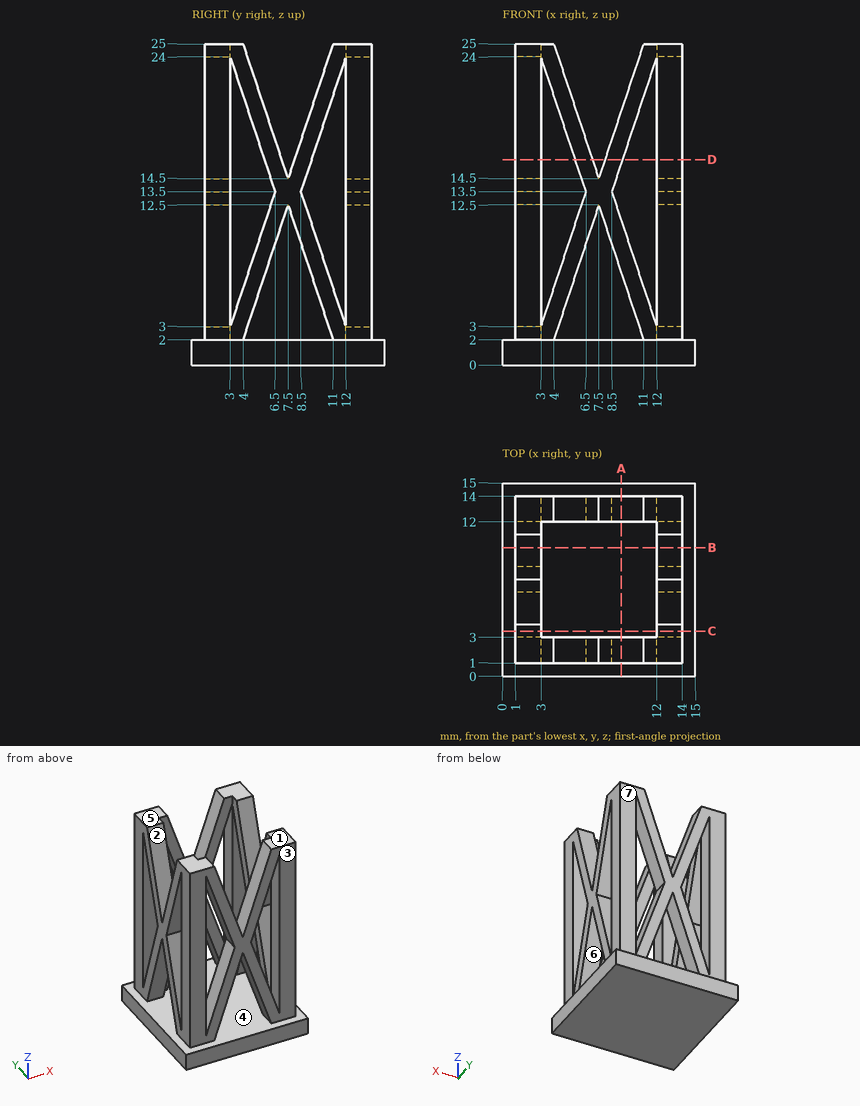
Input: dimensioned drawing with shaded views. Units: mm. Origin: part minimum x, y, z. A direction names the side the tool comes from. Round coordinates to 2 decimals unless told otherwise and drop trailing zeros. Loops run counter-clockwise (first coordinate to the right, second up) from the corner with the lowest first, then second, coordinate; pieces in that order, holes last. Notation, with made-up numbers: (-1, 56) -> (4, 56) arc R35 cw to (4, 88) -> close; hole circle Ø8 at (24, -34). An arc over 180 degrees is marked (long way). Use one line per item in the form item = value. Start each with the question number.
1) Section C-C on y = 3.5. Output: boundary loops of the cut face in (x, z), then the cut area to 3 significant figures.
2) Access query for the marked faces 1, 2, 3 and 4. Directions: +Z, -Z, +X, -X, +Y, -Y. A direction counts if a zero-diameter tool reaches every point of the face in a straight line with its end or side. Return the directions, or none.
3) Draft query along Y for the marked faces 5, 6 and 7. Return one class per face: released by +Y, released by -Y, zero draft, split by the parting line, or undercut.
4) Line query: L1, parallel to Y at x = 6, z = 11.25; L2, parallel to Y at x = 13.5, z = 5.5; L3, parallel to X at y = 2.5, z = 19.75. Output: solid intervals per line, ascending.
5) Section A-A on x = 9.25. Output: boundary loops of the cut face in (y, z).
6) Section D-D on z = 16. Give the number of separate pieces and of enclosed holes in the cut face, then the cut area to 3 significant figures.
7) First-contact query: P1, Ø8, axis at y = 12.5, z = 22, coming from the +X side; P2, Ø0.6, axis at y = 2.5, z = 13, coming from the -X side; P3, Ø6.5, axis at x = 10.5, z = 11, coming from the -Y side; P4, Ø8, axis at x = 8, y = 10, coming from the -Z side. Flat tips, straight axial feed; report the tip coordinate or a pass-through.
8) Section B-B on y = 10. Output: boundary loops of the cut face in (x, z), then the cut area to 3 significant figures.
Response:
q1.outline = (0, 0) -> (15, 0) -> (15, 2) -> (14, 2) -> (14, 4.5) -> (12, 4.5) -> (12, 2) -> (3, 2) -> (3, 4.5) -> (1, 4.5) -> (1, 2) -> (0, 2) -> close; (1, 22.5) -> (3, 22.5) -> (3, 25) -> (1, 25) -> close; (12, 22.5) -> (14, 22.5) -> (14, 25) -> (12, 25) -> close
q1.area = 50.0 mm^2
q2.face_1 = +Z, +X, -X, +Y, -Y
q2.face_2 = +Z, +X, -X
q2.face_3 = +Z, +X, -X, -Y
q2.face_4 = none
q3.face_5 = zero draft
q3.face_6 = undercut
q3.face_7 = released by +Y
q4.L1 = 1 to 3, 12 to 14
q4.L2 = 1 to 3, 3.83 to 5.17, 9.83 to 11.17, 12 to 14
q4.L3 = 1 to 3, 4.42 to 5.75, 9.25 to 10.58, 12 to 14
q5.outline = (0, 0) -> (15, 0) -> (15, 2) -> (0, 2) -> close; (1, 7.25) -> (3, 7.25) -> (3, 11.25) -> (1, 11.25) -> close; (1, 15.75) -> (3, 15.75) -> (3, 19.75) -> (1, 19.75) -> close; (12, 7.25) -> (14, 7.25) -> (14, 11.25) -> (12, 11.25) -> close; (12, 15.75) -> (14, 15.75) -> (14, 19.75) -> (12, 19.75) -> close
q6.separate_pieces = 12
q6.enclosed_holes = 0
q6.area = 37.3 mm^2
q7.P1 = 14
q7.P2 = 1
q7.P3 = 1
q7.P4 = 0
q8.outline = (0, 0) -> (15, 0) -> (15, 2) -> (0, 2) -> close; (1, 5) -> (3, 5) -> (3, 9) -> (1, 9) -> close; (1, 18) -> (3, 18) -> (3, 22) -> (1, 22) -> close; (12, 5) -> (14, 5) -> (14, 9) -> (12, 9) -> close; (12, 18) -> (14, 18) -> (14, 22) -> (12, 22) -> close
q8.area = 62.0 mm^2
